The model under review builds one solid part; all positions refer to its coordinate system, in mm. A direction names the side the tool comes from. Round coordinates to 2 decimals unless told otherwise and drop trailing zeros. Write each loop counter-clockwise with the first axis right and the second up, starting at its lowest first coordinate (ties: lowest second). Pieces come first, ordered by that corner, then holes. Notation, with made-up numbers: (17, 78) - (58, 78) arc R33 cw to (58, 112) - close; hole circle Ø6 at (6, 84.5). An arc over 180 degrees is marked (long way). Write each question's results on one line, items separated by ' | '.
```python
from build123d import *

# Parameters (mm, degrees)
SKETCH2_W           = 31.750972762
SKETCH2_H           = 30
BOSS_EXTRUDE1_DEPTH = 15
FILLET1_R           = 4
CHAMFER1_SIZE       = 3
CHAMFER2_SIZE       = 1
SKETCH4_R           = 10
BOSS_EXTRUDE2_DEPTH = 5
FILLET2_R           = 5
SKETCH5_W           = 5
SKETCH5_H           = 15
BOSS_EXTRUDE3_DEPTH = 20
CHAMFER3_SIZE       = 2
SKETCH6_R           = 5
CUT_EXTRUDE1_DEPTH  = 10
SKETCH7_R           = 0.75
BOSS_EXTRUDE4_DEPTH = 40
CIRPATTERN2_COUNT   = 8
SKETCH8_R           = 5
CUT_EXTRUDE2_DEPTH  = 10
CUT_EXTRUDE3_DEPTH  = 1
LPATTERN3_COUNT     = 2
LPATTERN3_PITCH     = 8
LPATTERN3_COL_COUNT = 2
LPATTERN3_COL_PITCH = 8


# Some blends are built 0.0001 mm under size
with BuildPart() as part:
    # Sketch2 → Boss-Extrude1 (new, symmetric)
    with BuildSketch(Plane.XY):
        Rectangle(SKETCH2_W, SKETCH2_H)
    extrude(amount=BOSS_EXTRUDE1_DEPTH, both=True)

    # Sketch3 → Revolve1 (revolve)
    with BuildSketch(Plane(origin=(0, 0, 0), x_dir=(0, 0, -1), z_dir=(1, 0, 0))):
        Polygon((-55, 0), (-55, 15), (-52, 15), (-52, 9), (-15, 9), (-15, 0), align=None)
    revolve(axis=Axis((0, 0, 15), (0, 0, 1)))

    # Fillet1
    fillet1_edges = [part.edges().sort_by_distance(p)[0] for p in [
        (15.875486381, -15, 0),
        (-15.875486381, -15, 0),
        (-15.875486381, 15, 0),
        (15.875486381, 15, 0),
    ]]
    fillet(fillet1_edges, radius=FILLET1_R)

    # Chamfer1
    # the kernel refuses this chamfer: 3 mm, written as the material it takes off along each edge
    with BuildSketch(Plane(origin=(15.875486381, 18.715048964, 15), x_dir=(-0.9996219169112969, 0, 0.02749587661058621), z_dir=(0, -1, 0))) as chamfer1_piece_1:
        Polygon((CHAMFER1_SIZE * 0.999621916911, CHAMFER1_SIZE * 0.0274958766106), (-CHAMFER1_SIZE * 0.0274958766106, CHAMFER1_SIZE * 0.999621916911), (0, 0), align=None)
    extrude(amount=37.430097928, mode=Mode.SUBTRACT)

    # Chamfer2
    chamfer2_edges = [part.edges().sort_by_distance(p)[0] for p in [
        (0, -15, -15),
        (14.703913506, -13.828427125, -15),
        (-14.703913506, -13.828427125, -15),
        (15.875486381, 0, -15),
        (-15.875486381, 0, -15),
        (14.703913506, 13.828427125, -15),
        (-14.703913506, 13.828427125, -15),
        (0, 15, -15),
        (12.379503551, -14.968118785, 15),
        (0, -15, 15),
        (-14.703913506, -13.828427125, 15),
        (-15.875486381, 0, 15),
        (12.379503551, 14.968118785, 15),
        (-14.703913506, 13.828427125, 15),
        (0, 15, 15),
    ]]
    chamfer(chamfer2_edges, length=CHAMFER2_SIZE)

    # Sketch4 → Boss-Extrude2 (add)
    with BuildSketch(Plane(origin=(0, 0, -15), x_dir=(-1, 0, 0), z_dir=(0, 0, -1))):
        Circle(SKETCH4_R)
    extrude(amount=BOSS_EXTRUDE2_DEPTH)

    # Fillet2
    fillet2_edges = [part.edges().sort_by_distance(p)[0] for p in [
        (10, 0, -20),
    ]]
    fillet(fillet2_edges, radius=FILLET2_R - 0.0001)  # a hair under: the kernel refuses the full size

    # Sketch5 → Boss-Extrude3 (add)
    with BuildSketch(Plane(origin=(0, 0, -15), x_dir=(-1, 0, 0), z_dir=(0, 0, -1))):
        with Locations((-15.875486381, 0)):
            Rectangle(SKETCH5_W, SKETCH5_H)
    extrude(amount=-BOSS_EXTRUDE3_DEPTH)

    # Chamfer3
    chamfer3_edges = [part.edges().sort_by_distance(p)[0] for p in [
        (18.375486381, 7.5, -5),
        (18.375486381, 0, 5),
        (18.375486381, -7.5, -5),
    ]]
    chamfer(chamfer3_edges, length=CHAMFER3_SIZE)

    # Sketch6 → Cut-Extrude1 (cut)
    with BuildSketch(Plane.XY.offset(55)):
        Circle(SKETCH6_R)
    extrude(amount=-CUT_EXTRUDE1_DEPTH, mode=Mode.SUBTRACT)

    # Sketch7 → Boss-Extrude4 (add)
    with BuildSketch(Plane.XY.offset(55)):
        with Locations((0, 11)):
            Circle(SKETCH7_R)
    boss_extrude4 = extrude(amount=-BOSS_EXTRUDE4_DEPTH)

    # CirPattern2: Boss-Extrude4 ×8 about axis
    cirpattern2_axis = Axis((0, 0, 0), (0, 0, 1))
    for i in range(1, CIRPATTERN2_COUNT):
        add(boss_extrude4.rotate(cirpattern2_axis, i * 360 / CIRPATTERN2_COUNT))

    # Sketch8 → Cut-Extrude2 (cut)
    with BuildSketch(Plane.ZY.offset(15.875486381)):
        Circle(SKETCH8_R)
    extrude(amount=-CUT_EXTRUDE2_DEPTH, mode=Mode.SUBTRACT)

    # Sketch9 → Cut-Extrude3 (cut)
    with BuildSketch(Plane(origin=(0, 15, 0), x_dir=(1, 0, 0), z_dir=(0, 1, 0))):
        with BuildLine():
            Line((1, 10), (1, -10))
            ThreePointArc((1, -10), (0, -11), (-1, -10))
            Line((-1, -10), (-1, 10))
            ThreePointArc((-1, 10), (0, 11), (1, 10))
        make_face()
    cut_extrude3 = extrude(amount=-CUT_EXTRUDE3_DEPTH, mode=Mode.SUBTRACT)

    # LPattern3: Cut-Extrude3 ×2
    with Locations(*[(-i * LPATTERN3_PITCH, 0, 0) for i in range(1, LPATTERN3_COUNT)]):
        add(cut_extrude3, mode=Mode.SUBTRACT)

    # LPattern3 col: Cut-Extrude3 ×2
    with Locations(*[(i * LPATTERN3_COL_PITCH, 0, 0) for i in range(1, LPATTERN3_COL_COUNT)]):
        add(cut_extrude3, mode=Mode.SUBTRACT)


solid = part.part
```
Q1. Insertion check: P1, Ø2, axis at y = -4, z = 38.5, coming from the +X side; P2, Ø0.5, axis at y = 14.5, z = -4, coming from the +X side; P3, Ø1.1, axis at y = 14.5, z = -3, coming from the -X side. Each pin has a flat end and moves straight along its axis. Give the tip position at first contact, or say it passes through.
Evaluation:
P1: stops at x = 8.49 | P2: stops at x = 14.21 | P3: stops at x = -14.58
Q2. For probe 1 along X at (y, z) = (0, 24.5); probe 2 along Y at (x, z) = (0, 47); probe 3 along Z at (x, y) = (7, 13), list the stretches that pass through material, from the lowest coordinate up.
Evaluation:
probe 1: x = -11.75 to -10.25, -9 to 9, 10.25 to 11.75 | probe 2: y = -11.75 to -10.25, -9 to -5, 5 to 9, 10.25 to 11.75 | probe 3: z = -15 to 15, 52 to 55
Q3. We need section C-C (x = -11). State the section outline as (y, z) points.
Evaluation:
outline: (-15, -14) - (-14, -15) - (14, -15) - (15, -14) - (15, 14) - (14, 15) - (0.75, 15) - (0.75, 52) - (10.2, 52) - (10.2, 55) - (-10.2, 55) - (-10.2, 52) - (-0.75, 52) - (-0.75, 15) - (-14, 15) - (-15, 14) - close; hole circle Ø10 at (0, 0)
Q4. The part is to be moulded in two halves that separate along Z. For faces 5 (the cylindrical face through (14.67, 13.86, -0.2)), 6 (the conical face through (-14.172, 13.348, 14.715)), 7 (the conical face through (-14.172, 13.348, -14.715)), 8 (the flat face through (6.5, 6.5, 52)), say which applies: released by +Z, released by -Z, zero draft, split by the parting line, or undercut.
Evaluation:
face 5: zero draft | face 6: released by +Z | face 7: released by -Z | face 8: undercut
Q5. We need section A-A (z = 20). State how many separate pieces and enclosed holes the cut face has, plus the area to 3 significant figures.
Evaluation:
separate pieces: 9 | enclosed holes: 0 | area: 269 mm^2
Q6. Tool access review of faces 1 (the cylindrical face through (-8.4, 8.2, 33.8)), 2 (the flat face through (-8, 14, 0)), 3 (the cylindrical face through (-10.95, -4.88, -1.08)), 4 (the flat face through (0, 0, 45)): name each direction out of +Z, -Z, +X, -X, +Y, -Y from which nothing blocks a thin tool from reaching the whole face with its end or side.
Evaluation:
face 1: none | face 2: +Y | face 3: -X | face 4: +Z
